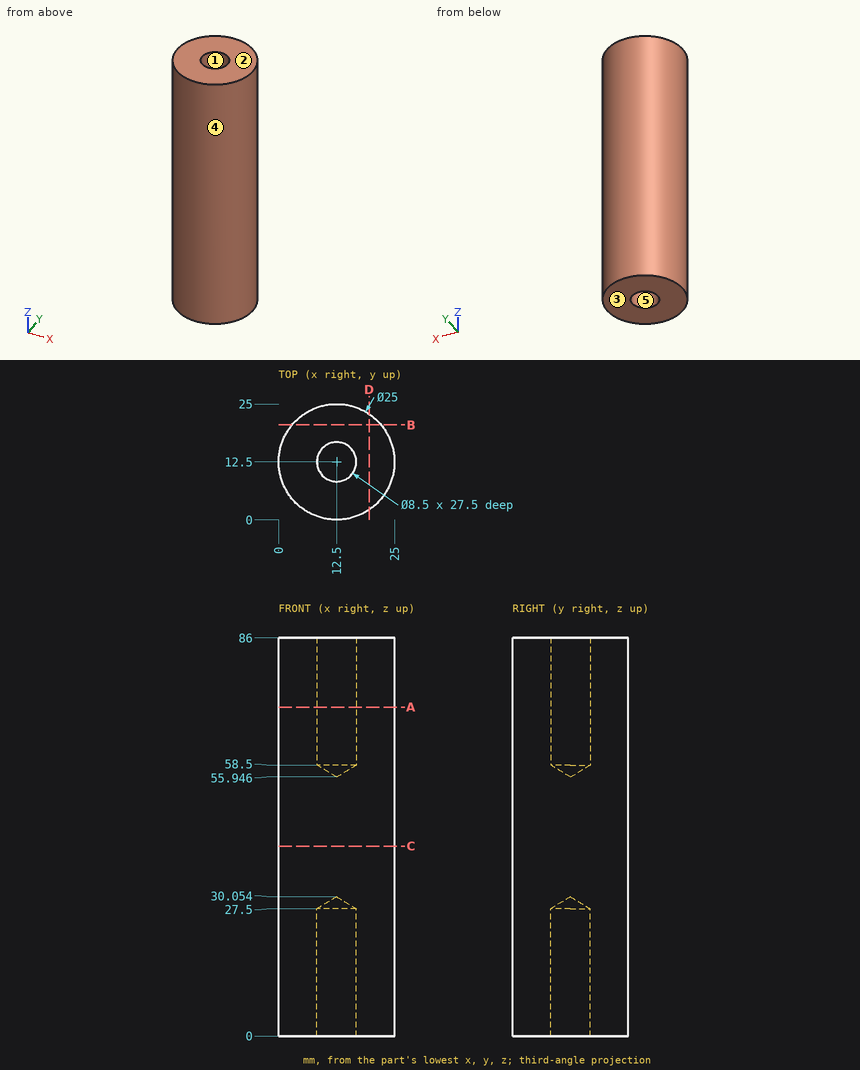
Here's the drawing with two shaded views (mm, measured from the low corner). I have some questions. A direction names the side the tool comes from. Coordinates: 2 decimals unless noted, no trailing zeros. Write each loop counter-clockwise with the first axis right and the second up, starting at its lowest first coordinate (ties: lowest second). Pieces come first, ordered by that corner, then holes. Notation, with made-up numbers: M 5,-9 L 45,-9 A23 ccw 45,7 Z; hole C 76,-10.75 d11. An arc over 180 degrees is marked long. Answer as CSV lines item,"result".
Item 1: We'd pull the mould along X, two halves only. Please class the marked faces 3, 4 and 5: +X half, -X half, draft (parallel to the pull), parting line (faces both ways), or undercut.
Geometry results:
face 3,"draft"
face 4,"parting line"
face 5,"undercut"
Item 2: Imagine slicing it at B-B on y = 20.5. List the corners of the cut face in (x, z) for me (1 decimal).
Geometry results:
outline,"M 2.9,0 L 22.1,0 L 22.1,86 L 2.9,86 Z"
Item 3: Imagine slicing it at D-D on x = 19.5. List the corners of the cut face in (y, z) for me.
Geometry results:
outline,"M 2.14,0 L 22.86,0 L 22.86,86 L 2.14,86 Z"
Item 4: Please list where these lines run through material, in increasing order: line 1 along X through (y, z) = (12.5, 74); line 2 along Y through (x, z) = (12, 8); line 3 along Y through (x, z) = (10.25, 63) (1 decimal).
Geometry results:
line 1,"x = 0 to 8.25, 16.75 to 25"
line 2,"y = 0.01 to 8.28, 16.72 to 24.99"
line 3,"y = 0.2 to 8.9, 16.1 to 24.8"
Item 5: On a 3-axis mill with a long thin cutter (end or side, diameter ignored), from which of +Z, -Z, +X, -X, +Y, -Y can I reach the whole of each face in a straight line? I mean the marked faces 1 and 2. Say none if no direction works.
Geometry results:
face 1,"+Z"
face 2,"+Z, +X, -X, +Y, -Y"
Item 6: I'm going to push flat-ended pins straight in: P1, Ø1, axis at x = 14.5, z = 25.5, coming from the +Y side; P2, Ø3, axis at y = 2.5, z = 30.5, coming from the -X side (1 decimal); P3, Ø7, axis at x = 12.5, y = 12.5, coming from the +Z side. Where does each tip first touch, or does it pass through?
Geometry results:
P1,"stops at y = 24.91"
P2,"stops at x = 3.3"
P3,"stops at z = 58.05"
Item 7: Imagine slicing it at C-C on z = 41. List the corners of the cut face in (x, y) for me, plus the area to 3 significant figures.
Geometry results:
outline,"C 12.5,12.5 d25"
area,"491 mm2"
Item 8: Imagine slicing it at A-A on z = 71. List the corners of the cut face in (x, y) for me, plus the area to 3 significant figures.
Geometry results:
outline,"C 12.5,12.5 d25; hole C 12.5,12.5 d8.5"
area,"434 mm2"
